For this review, take the finished solid that the model builds, in its own axes (mm). Face numbers are marked on the shaded views. A direction names the side the tool comes from. Coordinates: 2 decimals unless noted, no trailing zeros. Write each loop counter-clockwise with the first axis right and the second up, starting at its lowest first coordinate (ties: lowest second). Pieces come first, ordered by that corner, then holes. Notation, with made-up numbers: M -25,1.5 L -2,1.5 A19 ccw -2,36.5 Z; hole C 85,6.5 d4. An arc over 180 degrees is marked long. One line per question, with ' | ' between items.
from build123d import *

# Parameters (mm, degrees)
BOSS_EXTRUDE1_DEPTH = 17.5
CUT_EXTRUDE1_REACH  = 85.725
SKETCH2_R           = 0.75
SKETCH2_3_R         = 0.75
CUT_EXTRUDE2_DEPTH  = 84.724608091


with BuildPart() as part:
    # Sketch1 → Boss-Extrude1 (new, symmetric)
    with BuildSketch(Plane(origin=(0, 0, 0), x_dir=(1, 0, 0), z_dir=(0, 1, 0))):
        with BuildLine():
            Line((-29.2, 0), (29.2, 0))
            ThreePointArc((29.2, 0), (32.735533906, 1.464466094), (34.2, 5))
            Line((34.2, 5), (34.2, 45))
            Line((34.2, 45), (30.7, 45))
            Line((30.7, 45), (30.7, 10))
            ThreePointArc((30.7, 10), (29.235533906, 6.464466094), (25.7, 5))
            Line((25.7, 5), (-25.7, 5))
            ThreePointArc((-25.7, 5), (-29.235533906, 6.464466094), (-30.7, 10))
            Line((-30.7, 10), (-30.7, 45))
            Line((-30.7, 45), (-34.2, 45))
            Line((-34.2, 45), (-34.2, 5))
            ThreePointArc((-34.2, 5), (-32.735533906, 1.464466094), (-29.2, 0))
        make_face()
    extrude(amount=BOSS_EXTRUDE1_DEPTH, both=True)

    # Cut-Extrude1: up to this face of the body (flat: up to its plane)
    cut_extrude1_end = Plane(part.part.faces().sort_by_distance((34.2, 0, -25))[0])
    # Sketch2 → Cut-Extrude1 (cut, up to the picked face)
    with BuildSketch(Plane.ZY.offset(34.2), mode=Mode.PRIVATE) as cut_extrude1_sk1:
        with Locations((-27, 12.5)):
            Circle(SKETCH2_R)
    cut_extrude1_tool1 = split(extrude(cut_extrude1_sk1.sketch, amount=-CUT_EXTRUDE1_REACH, mode=Mode.PRIVATE), bisect_by=cut_extrude1_end, keep=Keep.BOTH, mode=Mode.PRIVATE)
    # Sketch2 → Cut-Extrude1 (cut, up to the picked face)
    with BuildSketch(Plane.ZY.offset(34.2), mode=Mode.PRIVATE) as cut_extrude1_sk2:
        with Locations((-18.161165235, 8.838834765)):
            Circle(SKETCH2_R)
    cut_extrude1_tool2 = split(extrude(cut_extrude1_sk2.sketch, amount=-CUT_EXTRUDE1_REACH, mode=Mode.PRIVATE), bisect_by=cut_extrude1_end, keep=Keep.BOTH, mode=Mode.PRIVATE)
    # Sketch2 → Cut-Extrude1 (cut, up to the picked face)
    with BuildSketch(Plane.ZY.offset(34.2), mode=Mode.PRIVATE) as cut_extrude1_sk3:
        with Locations((-14.5, 0)):
            Circle(SKETCH2_R)
    cut_extrude1_tool3 = split(extrude(cut_extrude1_sk3.sketch, amount=-CUT_EXTRUDE1_REACH, mode=Mode.PRIVATE), bisect_by=cut_extrude1_end, keep=Keep.BOTH, mode=Mode.PRIVATE)
    # Sketch2 → Cut-Extrude1 (cut, up to the picked face)
    with BuildSketch(Plane.ZY.offset(34.2), mode=Mode.PRIVATE) as cut_extrude1_sk4:
        with Locations((-18.161165235, -8.838834765)):
            Circle(SKETCH2_R)
    cut_extrude1_tool4 = split(extrude(cut_extrude1_sk4.sketch, amount=-CUT_EXTRUDE1_REACH, mode=Mode.PRIVATE), bisect_by=cut_extrude1_end, keep=Keep.BOTH, mode=Mode.PRIVATE)
    # Sketch2 → Cut-Extrude1 (cut, up to the picked face)
    with BuildSketch(Plane.ZY.offset(34.2), mode=Mode.PRIVATE) as cut_extrude1_sk5:
        with Locations((-35.838834765, -8.838834765)):
            Circle(SKETCH2_R)
    cut_extrude1_tool5 = split(extrude(cut_extrude1_sk5.sketch, amount=-CUT_EXTRUDE1_REACH, mode=Mode.PRIVATE), bisect_by=cut_extrude1_end, keep=Keep.BOTH, mode=Mode.PRIVATE)
    # Sketch2 → Cut-Extrude1 (cut, up to the picked face)
    with BuildSketch(Plane.ZY.offset(34.2), mode=Mode.PRIVATE) as cut_extrude1_sk6:
        with Locations((-39.5, 0)):
            Circle(SKETCH2_R)
    cut_extrude1_tool6 = split(extrude(cut_extrude1_sk6.sketch, amount=-CUT_EXTRUDE1_REACH, mode=Mode.PRIVATE), bisect_by=cut_extrude1_end, keep=Keep.BOTH, mode=Mode.PRIVATE)
    # Sketch2 → Cut-Extrude1 (cut, up to the picked face)
    with BuildSketch(Plane.ZY.offset(34.2), mode=Mode.PRIVATE) as cut_extrude1_sk7:
        with Locations((-35.838834765, 8.838834765)):
            Circle(SKETCH2_R)
    cut_extrude1_tool7 = split(extrude(cut_extrude1_sk7.sketch, amount=-CUT_EXTRUDE1_REACH, mode=Mode.PRIVATE), bisect_by=cut_extrude1_end, keep=Keep.BOTH, mode=Mode.PRIVATE)
    add(cut_extrude1_tool1.solids().sort_by(Axis((-34.2, 12.5, -27), (1, 0, 0)))[0], mode=Mode.SUBTRACT)
    add(cut_extrude1_tool2.solids().sort_by(Axis((-34.2, 8.838835, -18.161165), (1, 0, 0)))[0], mode=Mode.SUBTRACT)
    add(cut_extrude1_tool3.solids().sort_by(Axis((-34.2, 0, -14.5), (1, 0, 0)))[0], mode=Mode.SUBTRACT)
    add(cut_extrude1_tool4.solids().sort_by(Axis((-34.2, -8.838835, -18.161165), (1, 0, 0)))[0], mode=Mode.SUBTRACT)
    add(cut_extrude1_tool5.solids().sort_by(Axis((-34.2, -8.838835, -35.838835), (1, 0, 0)))[0], mode=Mode.SUBTRACT)
    add(cut_extrude1_tool6.solids().sort_by(Axis((-34.2, 0, -39.5), (1, 0, 0)))[0], mode=Mode.SUBTRACT)
    add(cut_extrude1_tool7.solids().sort_by(Axis((-34.2, 8.838835, -35.838835), (1, 0, 0)))[0], mode=Mode.SUBTRACT)

    # Sketch2<3> → Cut-Extrude2 (cut, through all)
    with BuildSketch(Plane.ZY.offset(34.2)):
        with Locations((-27, -12.5)):
            Circle(SKETCH2_3_R)
    extrude(amount=-CUT_EXTRUDE2_DEPTH, mode=Mode.SUBTRACT)


solid = part.part
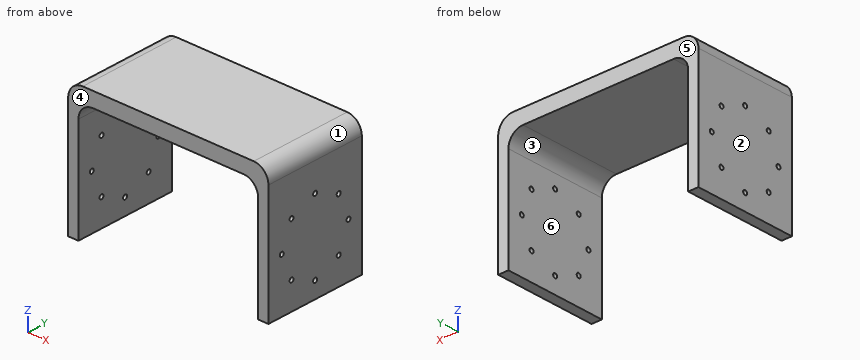
1. Take a section at A-A on z = -38. State the section outline as (x, y) points, plus the area to 3 significant figures.
Computed values:
outline: M -34.2,-17.5 L -30.7,-17.5 L -30.7,17.5 L -34.2,17.5 Z; M 30.7,-17.5 L 34.2,-17.5 L 34.2,17.5 L 30.7,17.5 Z | area: 245 mm2
2. Take a section at B-B on y = 0. State the section outline as (x, z) points, plus the area to 3 significant figures.
Computed values:
outline: M -34.2,-45 L -30.7,-45 L -30.7,-40.25 L -34.2,-40.25 Z; M -34.2,-38.75 L -30.7,-38.75 L -30.7,-15.25 L -34.2,-15.25 Z; M -34.2,-13.75 L -30.7,-13.75 L -30.7,-10 A5 cw -25.7,-5 L 25.7,-5 A5 cw 30.7,-10 L 30.7,-13.75 L 34.2,-13.75 L 34.2,-5 A5 ccw 29.2,0 L -29.2,0 A5 ccw -34.2,-5 Z; M 30.7,-45 L 34.2,-45 L 34.2,-40.25 L 30.7,-40.25 Z; M 30.7,-38.75 L 34.2,-38.75 L 34.2,-15.25 L 30.7,-15.25 Z | area: 601 mm2
3. For line 1 along Y through (x, z) = (-33, -27); line 2 along X through (y, z) = (-9, -41.5); line 3 along Z through (x, y) = (-13, 3), list the stretches that pass through material, from the lowest coordinate up.
Computed values:
line 1: y = -17.5 to -13.25, -11.75 to 11.75, 13.25 to 17.5 | line 2: x = -34.2 to -30.7, 30.7 to 34.2 | line 3: z = -5 to 0
4. Draft analysis for pull direction X (two halves, no side actions). For the marked faces 1, 2, 3 and 4, state which applies: pulls with the +X half, pulls with the -X half, needs draft (parallel to the pull), parting line crosses it, or undercut.
Computed values:
face 1: pulls with the +X half | face 2: pulls with the -X half | face 3: undercut | face 4: needs draft
5. Clearance check with flat-ended pins moving along their axes: P1, Ø0.9, axis at y = 0, z = -39.5, coming from the -X side; P2, Ø1.5, axis at x = 21.5, y = 11, coming from the -Z side. State where each tip first meets the part, or that it passes through.
Computed values:
P1: passes through | P2: stops at z = -5
6. Take a section at D-D on y = 12.5. State the section outline as (x, z) points.
Computed values:
outline: M -34.2,-45 L -30.7,-45 L -30.7,-27.75 L -34.2,-27.75 Z; M -34.2,-26.25 L -30.7,-26.25 L -30.7,-10 A5 cw -25.7,-5 L 25.7,-5 A5 cw 30.7,-10 L 30.7,-26.25 L 34.2,-26.25 L 34.2,-5 A5 ccw 29.2,0 L -29.2,0 A5 ccw -34.2,-5 Z; M 30.7,-45 L 34.2,-45 L 34.2,-27.75 L 30.7,-27.75 Z
7. Machinability: for the marked faces 5 and 6, which of the approach directions +Z, -Z, +X, -X, +Y, -Y give a long, thin tool a straight path to every point of the face, cutting with its end or side? Answer none if there is none.
Computed values:
face 5: +Z, -Z, +X, -X, +Y | face 6: -Z, +Y, -Y
8. Take a section at C-C on z = -14.5. State the section outline as (x, y) points, plus the area to 4 significant figures.
Computed values:
outline: M -34.2,-17.5 L -30.7,-17.5 L -30.7,-0.75 L -34.2,-0.75 Z; M -34.2,0.75 L -30.7,0.75 L -30.7,17.5 L -34.2,17.5 Z; M 30.7,-17.5 L 34.2,-17.5 L 34.2,-0.75 L 30.7,-0.75 Z; M 30.7,0.75 L 34.2,0.75 L 34.2,17.5 L 30.7,17.5 Z | area: 234.5 mm2
